For this review, take the finished solid that the model builds, in its own axes (mm). Face numbers are marked on the shaded views. A direction names the side the tool comes from. Coordinates: 2 decimals unless noted, no trailing zeros. Order: outer loops, then holes, each group sorted by start corner. A loop starts at its lowest first (then second) coordinate and runs counter-clockwise, first axis right, second up. Notation, with made-up numbers: M 44.25,82.5 L 98.25,82.5 A14 cw 98.25,93.5 Z; hole C -4.5,-6.75 d9. An arc over 180 degrees is marked long. Use CSV: the item, a comma, the result in double quotes.
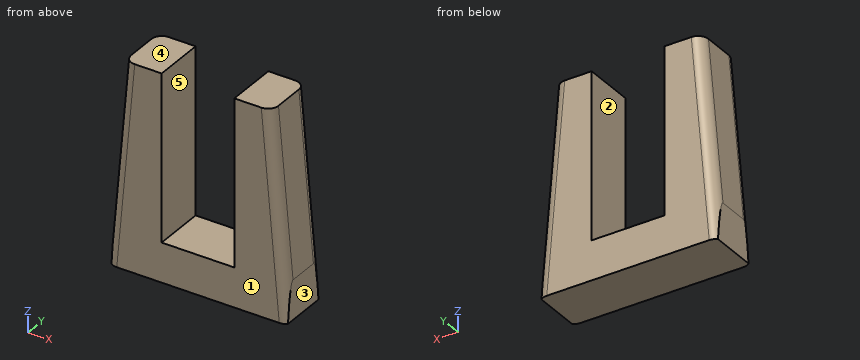
```python
from build123d import *

# Parameters (mm, degrees)
F1_DEPTH    = 2.5
F2_T1_DEPTH = 15.5305666052
F2_T3_DEPTH = 15.5305666052


# Not quite as in the source:
# - a fillet or chamfer that OpenCascade refuses, or shapes differently, is made with other operations: its cross-section is extruded or revolved along the edge and cut away or added


with BuildPart() as f1:
    # F0 (on Front) → F1 (new body)
    with BuildSketch(Plane.XZ):
        Polygon((0, -1.894692351), (0, 0), (-1.75, 0), (-4.25, 0), (-4.25, -1.894692351), align=None)
        Polygon((1.75, 0), (0, 0), (0, -1.894692351), (4.25, -1.894692351), (4.25, 0), align=None)
        Polygon((-4.25, 0), (-1.75, 0), (-1.75, 8), (-3.55, 8), align=None)
        Polygon((1.75, 8), (1.75, 0), (4.25, 0), (3.55, 8), align=None)
    extrude(amount=F1_DEPTH)

    # F2: fillet of radius 0.5 on 4 edges, made by hand

    # F2_s2 → F2_t1 (cut)
    with BuildSketch(Plane(origin=(0.5770852674, 0, -6.5952601994), x_dir=(0, 1, 0), z_dir=(-0.0871669503, 0, 0.9961937175))):
        with BuildLine():
            ThreePointArc((-2, -4.2338232994), (-2.3535533906, -4.08737669), (-2.5, -3.7338232994))
            Line((-2.5, -3.7338232994), (-2.5, -4.2338232994))
            Line((-2.5, -4.2338232994), (-2, -4.2338232994))
        make_face()
        with BuildLine():
            ThreePointArc((-0.5, -4.2338232994), (-0.1464466094, -4.08737669), (0, -3.7338232994))
            Line((0, -3.7338232994), (0, -4.2338232994))
            Line((0, -4.2338232994), (-0.5, -4.2338232994))
        make_face()
    extrude(amount=F2_T1_DEPTH, mode=Mode.SUBTRACT)

    # F2_s4 → F2_t3 (cut)
    with BuildSketch(Plane(origin=(0.7766668597, 0, 8.8761926818), x_dir=(0, 1, 0), z_dir=(-0.0871669503, 0, -0.9961937175))):
        with BuildLine():
            ThreePointArc((-2, -4.2338232994), (-2.3535533906, -4.08737669), (-2.5, -3.7338232994))
            Line((-2.5, -3.7338232994), (-2.5, -4.2338232994))
            Line((-2.5, -4.2338232994), (-2, -4.2338232994))
        make_face()
        with BuildLine():
            ThreePointArc((-0.5, -4.2338232994), (-0.1464466094, -4.08737669), (0, -3.7338232994))
            Line((0, -3.7338232994), (0, -4.2338232994))
            Line((0, -4.2338232994), (-0.5, -4.2338232994))
        make_face()
    extrude(amount=F2_T3_DEPTH, mode=Mode.SUBTRACT)


solid = f1.part
```
Item 1: Draft analysis for pull direction X (two halves, no side actions). For the marked faces 1, 2 and 3, state which applies: released by +X, released by -X, zero draft, split by the parting line, or undercut.
Solutions:
face 1,"zero draft"
face 2,"undercut"
face 3,"released by +X"
Item 2: To check wall thickness, follow line 1 along Z through (x, y) = (-1.25, -1.6); line 2 along Y through (x, z) = (3.5, 3.5); line 3 along X through (y, z) = (-1.1, 2.75). State the ranges of each line that lie inside material, in increasing order. Write a range as [from, to].
Solutions:
line 1,"[-1.89, 0]"
line 2,"[-2.5, 0]"
line 3,"[-4.01, -1.75], [1.75, 4.01]"
Item 3: For the marked faces 4 and 5, list the 3-axis set-ups (+Z, -Z, +X, -X, +Y, -Y) from which the entire face can be reached by the end or side of a thin tool; tool diameter is ignored.
Solutions:
face 4,"+Z, +X, -X, +Y, -Y"
face 5,"+Z, +Y, -Y"
Item 4: Add section A-A on y = -0.7. State the section outline as (x, z) points, and give its area (3 significant figures).
Solutions:
outline,"M -4.25,-1.89 L 4.25,-1.89 L 4.25,0 L 3.55,8 L 1.75,8 L 1.75,0 L -1.75,0 L -1.75,8 L -3.55,8 L -4.25,0 Z"
area,"50.5 mm^2"
Item 5: Add section C-C on y = -2.2. State the section outline as (x, z) points, and give its area (3 significant figures).
Solutions:
outline,"M -4.25,-1.89 L 4.25,-1.89 L 4.25,-0.48 L 3.51,8 L 1.75,8 L 1.75,0 L -1.75,0 L -1.75,8 L -3.51,8 L -4.25,-0.48 Z"
area,"49.8 mm^2"
Item 6: Add section B-B on x = -1.25. State the section outline as (y, z) points, and give its area (3 significant figures).
Solutions:
outline,"M -2.5,-1.89 L 0,-1.89 L 0,0 L -2.5,0 Z"
area,"4.74 mm^2"
Item 7: Clearance check with a flat-ended pin moving along its axis: pin 1 Ø1.5 at (y, z) = (-0.5, 4) entering from -X. State where the tip first meets the part, or that it passes through.
Solutions:
pin 1,"x = -3.97"
